from build123d import *

# Parameters (mm, degrees)
CHAMFER1_SIZE = 4


with BuildPart() as part:
    # Sketch1 → Revolve1 (revolve)
    with BuildSketch(Plane.XY):
        Polygon((1.4, 0), (1.4, 36.5), (10, 36.5), (10, 30.5), (6, 30.5), (6, 6), (10, 6), (10, 0), align=None)
    revolve(axis=Axis((0, -42.821890518, 0), (0, 1, 0)))

    # Chamfer1
    chamfer1_edges = [part.edges().sort_by_distance(p)[0] for p in [
        (-6, 6, 0),
        (-6, 30.5, 0),
    ]]
    chamfer(chamfer1_edges, length=CHAMFER1_SIZE - 0.0001)  # a hair under: the kernel refuses the full size


solid = part.part
The listing builds one solid part. Answer for the finished solid, in the listing's coordinates (mm). A direction names the side the tool comes from. Round coordinates to 2 decimals unless told otherwise and drop trailing zeros. Write each question's results on one line, items separated by ' | '. Start each with the question number.
Q1. Straight lines are drawn through the part: probe 1 along X at (y, z) = (20, 0); probe 2 along X at (y, z) = (8.5, 0). For each, find the intervals that lie inside material, in ascending order. Write a range as from..to.
Q2. Which of the six approach directions +Z, -Z, +X, -X, +Y, -Y give full straight-line access (tool end or side, diameter ignored) to faces 1 (the cylindrical face through (-1.4, 18.51, -0.06)), 2 (the cylindrical face through (-6, 18, 0))?
Q3. Each of these flat-tipped pins is pushed along its axis until it touches: pin 1 (6 mm diameter, centred on x = -7.5, y = 11.5, fed in from -Z); pin 2 (1 mm diameter, centred on y = 15.5, z = 3, fed in from +X); pin 3 (2 mm diameter, centred on y = 16.5, z = 0, fed in from +X); pin 4 (2 mm diameter, centred on x = 0, z = 0, fed in from +Y). Where does it stop, or does it pass through?
Q4. The mould has two halves that part along Y. Classify faces 3 (the flat face through (2, 0, 0)), 4 (the conical face through (5.96, 9.75, -1.88)), 5 (the cylindrical face through (-2.17, 2.96, 9.76)), 6 (the conical face through (-4.9, 26.7, 3.8)): pulls with the +Y half, pulls with the -Y half, needs draft (parallel to the pull), parting line crosses it, or undercut.
Worked answers:
1) probe 1: x = -6..-1.4, 1.4..6 | probe 2: x = -7.5..-1.4, 1.4..7.5
2) face 1: +Y, -Y | face 2: none
3) pin 1: stops at z = -3.97 | pin 2: stops at x = 5.45 | pin 3: stops at x = 6 | pin 4: passes through
4) face 3: pulls with the -Y half | face 4: undercut | face 5: needs draft | face 6: undercut
